Read the model definition and answer for the solid it produces. Units are mm, in the model's axes. Face numbers are marked on the shaded views. Give positions to 0.01 mm unless a question says otherwise; leave off trailing zeros. Order: outer loops, then holes, each group sorted by start corner. A loop starts at its lowest first (then second) coordinate and runs counter-clockwise, first axis right, second up. Notation, with made-up numbers: M 38.5,-18 L 60.5,-18 A17 cw 60.5,13 Z; hole C -33.5,11.25 d7. An arc over 180 degrees is marked long. One line per item, written item: value.
from build123d import *

# Parameters (mm, degrees)
F0_W     = 75
F0_H     = 50
F0_W_2   = 71
F0_H_2   = 46
F1_DEPTH = 970
F3_R     = 2
F4_R     = 2
F2_W     = 69
F2_H     = 100
F5_DEPTH = 60


with BuildPart() as f1:
    # F0 (on Front) → F1 (new body)
    with BuildSketch(Plane.XZ):
        Rectangle(F0_W, F0_H)
        Rectangle(F0_W_2, F0_H_2, mode=Mode.SUBTRACT)
    extrude(amount=F1_DEPTH)

    # F3
    f3_edges = [f1.edges().sort_by_distance(p)[0] for p in [
        (-37.5, -485, 25),
        (37.5, -485, 25),
        (37.5, -485, -25),
        (-37.5, -485, -25),
    ]]
    fillet(f3_edges, radius=F3_R)

    # F4
    f4_edges = [f1.edges().sort_by_distance(p)[0] for p in [
        (-35.5, -485, 23),
        (-35.5, -485, -23),
        (35.5, -485, -23),
        (35.5, -485, 23),
    ]]
    fillet(f4_edges, radius=F4_R)

    # F2 (on face) → F5 (cut)
    with BuildSketch(Plane.XY.offset(25)):
        with Locations((-0.465244, -814.95)):
            Rectangle(F2_W, F2_H)
        with Locations((-0.465244, -662.64)):
            Rectangle(F2_W, F2_H)
        with Locations((-0.465244, -510.33)):
            Rectangle(F2_W, F2_H)
        with Locations((-0.465244, -358.02)):
            Rectangle(F2_W, F2_H)
        with Locations((-0.465244, -205.71)):
            Rectangle(F2_W, F2_H)
        with Locations((-0.465244, -53.4)):
            Rectangle(F2_W, F2_H)
    extrude(amount=-F5_DEPTH, mode=Mode.SUBTRACT)


solid = f1.part
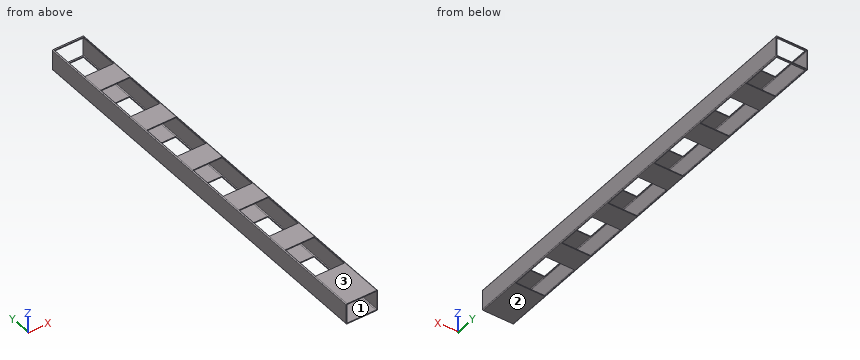
1) Find section C-C, the plane x = 14. Count the separate pieces of the cut face and the enclosed holes in it, plus the area to 3 significant figures.
Reported:
separate pieces: 14
enclosed holes: 0
area: 1,480 mm^2
2) Consider probe 1 along X at (y, z) = (-405, -2); probe 2 along Z at (x, y) = (5.5, -759.5); probe 3 along X at (y, z) = (-718.5, 22). Determine where each line is inside the solid, lowest interval first.
Reported:
probe 1: x = -37.5 to -35.5, 35.5 to 37.5
probe 2: z = -25 to -23, 23 to 25
probe 3: x = -37.5 to -35.23, 35.23 to 37.5
3) Find section D-D, the plane y = -892.5. Write down the section's boundary in (x, z).
Reported:
outline: M -37.5,-23 A2 ccw -35.5,-25 L 35.5,-25 A2 ccw 37.5,-23 L 37.5,23 A2 ccw 35.5,25 L -35.5,25 A2 ccw -37.5,23 Z; hole M -35.5,-21 A2 ccw -33.5,-23 L 33.5,-23 A2 ccw 35.5,-21 L 35.5,21 A2 ccw 33.5,23 L -33.5,23 A2 ccw -35.5,21 Z
4) Determine the mould class of the marked faces 1, 2 and 3 for opening direction Z: +Z half, -Z half, draft (parallel to the pull), parting line (faces both ways), or undercut.
Reported:
face 1: undercut
face 2: -Z half
face 3: +Z half
5) Find section B-B, the plane y = -776. Write down the section's boundary in (x, z).
Reported:
outline: M -37.5,-23 A2 ccw -35.5,-25 L -34.97,-25 L -34.97,-22.36 A2 cw -35.5,-21 L -35.5,21 A2 cw -34.97,22.36 L -34.97,25 L -35.5,25 A2 ccw -37.5,23 Z; M 34.03,-25 L 35.5,-25 A2 ccw 37.5,-23 L 37.5,23 A2 ccw 35.5,25 L 34.03,25 L 34.03,22.93 A2 cw 35.5,21 L 35.5,-21 A2 cw 34.03,-22.93 Z
6) Each of these flat-tipped pins is pushed along its axis until it touches: pin 1 Ø0.6 at (y, z) = (-839, 24.5) entering from -X; pin 2 Ø0.6 at (y, z) = (-359.5, 24) entering from -X; pin 3 Ø1 at (y, z) = (-523.5, 24.5) entering from -X. Where does it stop, or does it pass through?
Reported:
pin 1: stops at x = -37.1
pin 2: stops at x = -37.37
pin 3: stops at x = -37.23
7) Find section A-A, the plane z = -8. Write down the section's boundary in (x, y), plus the area to 3 significant figures.
Reported:
outline: M -37.5,-970 L -35.5,-970 L -35.5,0 L -37.5,0 Z; M 35.5,-970 L 37.5,-970 L 37.5,0 L 35.5,0 Z
area: 3,880 mm^2
